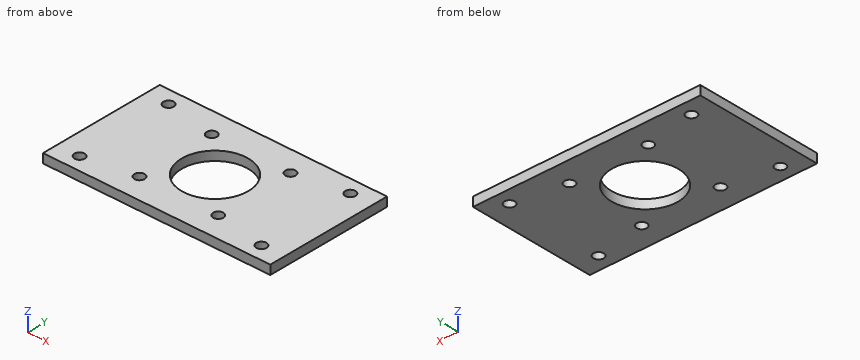
from build123d import *

# Parameters (mm, degrees)
SKETCH1_W            = 75
SKETCH1_H            = 42
BOSS_EXTRUDE1_DEPTH  = 3
SKETCH2_R            = 11
CUT_EXTRUDE1_DEPTH   = 4
M3_CLEARANCE_HOLE1_D = 3.4
M3_CLEARANCE_HOLE2_D = 3.4


with BuildPart() as part:
    # Sketch1 → Boss-Extrude1 (new body)
    with BuildSketch(Plane.XY):
        Rectangle(SKETCH1_W, SKETCH1_H)
    extrude(amount=BOSS_EXTRUDE1_DEPTH)

    # Sketch2 → Cut-Extrude1 (cut, through all)
    with BuildSketch(Plane.XY.offset(3)):
        Circle(SKETCH2_R)
    extrude(amount=-CUT_EXTRUDE1_DEPTH, mode=Mode.SUBTRACT)

    # M3 Clearance Hole1 (through all)
    with Locations(Plane.XY.offset(3)):
        with Locations((-13, -13), (13, -13), (13, 13), (-13, 13)):
            Hole(M3_CLEARANCE_HOLE1_D / 2)

    # M3 Clearance Hole2 (through all)
    with Locations(Plane.XY.offset(3)):
        with Locations((-30, -16), (-30, 16), (30, -16), (30, 16)):
            Hole(M3_CLEARANCE_HOLE2_D / 2)


solid = part.part
Part model, mm, in its own coordinate system. Coordinates: 2 decimals unless noted, no trailing zeros. Loops run counter-clockwise (first coordinate to the right, second up) from the corner with the lowest first, then second, coordinate; pieces in that order, holes last. Notation, with made-up numbers: (86, -5) - (119, -5) arc R23 cw to (119, 29) - close; hole circle Ø10 at (74.25, -35.75). An arc over 180 degrees is marked (long way). Write each question's results on one line, items separated by ' | '. Start each with the question number.
Q1. Probe line 1 along Y through (x, z) = (30, 1.8); line 2 along Y through (x, z) = (-13, 1.35); line 3 along X through (y, z) = (-15, 1.3). List the from-to ranges inside material, lowest first.
Q2. Drop a flat-ended pin along its axis: pin 1 Ø3 at (x, y) = (-13, -13) entering from +Z. Give the stop position or say it passes through.
Q3. Slice it at B-B on x = 0. Give the cut face in (y, z), and give its area (3 significant figures).
Q4. Slice it at C-C on z = 1.75. Give the number of separate pieces and of enclosed holes in the cut face, and give its area (3 significant figures).
Q5. Slice it at A-A on y = -13. Give the cut face in (x, z).
Q6. Slice it at D-D on y = 0. Give the cut face in (x, z).
Answer:
1) line 1: y = -21 to -17.7, -14.3 to 14.3, 17.7 to 21 | line 2: y = -21 to -14.7, -11.3 to 11.3, 14.7 to 21 | line 3: x = -37.5 to -31.37, -28.63 to 28.63, 31.37 to 37.5
2) pin 1: passes through
3) outline: (-21, 0) - (-11, 0) - (-11, 3) - (-21, 3) - close; (11, 0) - (21, 0) - (21, 3) - (11, 3) - close | area: 60.0 mm2
4) separate pieces: 1 | enclosed holes: 9 | area: 2,700 mm2
5) outline: (-37.5, 0) - (-14.7, 0) - (-14.7, 3) - (-37.5, 3) - close; (-11.3, 0) - (11.3, 0) - (11.3, 3) - (-11.3, 3) - close; (14.7, 0) - (37.5, 0) - (37.5, 3) - (14.7, 3) - close
6) outline: (-37.5, 0) - (-11, 0) - (-11, 3) - (-37.5, 3) - close; (11, 0) - (37.5, 0) - (37.5, 3) - (11, 3) - close
